Can you work these out from the model? Positions are in its coordinate system, mm. A direction names the side the tool comes from. Round coordinates to 2 decimals unless told otherwise and drop trailing zeros. Loops run counter-clockwise (first coordinate to the right, second up) from the corner with the lowest first, then second, coordinate; pieces in that order, holes last.
(1) If I drill on line 1 along Y through (x, z) = (-34, -19); line 2 along Y through (x, z) = (-16, -17); line 3 along Z through (x, y) = (-27.5, 6.5), over which ranges is the centre line in solid material (lowest first)?
(2) Which directions (+Z, -Z, +X, -X, +Y, -Y) give clear straight access to the entire face, cutting with the end or side of a thin tool? Please do faces 5 (the face through (8.428, 50.42, 1.107)), 6 (the face through (33, 2, 21)), 7 (the face through (39.05, 8.99, 8.67)).
(3) Thinking about a two-plate mould opening in Y: for faces 1 (the face through (0.33, 87.014, -7.493)), 2 (the face through (-14.75, 4.96, 35.58)), 3 (the face through (-3.874, 82.958, -5.052)), 4 (the face through (1, 0, 1)), which applies, released by +Y, released by -Y, zero draft, split by the parting line, or undercut?
(4) Will these pins go through, and if not, where does the flat tip stop? pin 1 Ø24 at (x, z) = (9.5, 15) entering from -Y; pin 2 Ø8 at (y, z) = (66, -3) entering from -X; pin 3 Ø12 at (y, z) = (57.5, 5) entering from +X; pin 4 Ø8 at (y, z) = (19, 11) entering from +X.
(5) I want a section at C-C on y = 23.5. Write out the boundary of the cut face in (x, z), plus the area to 3 significant figures.
(6) I want a section at D-D on z = 26. Write out the boundary of the cut face in (x, y), plus the area to 3 significant figures.
from build123d import *

# Parameters (mm, degrees)
SKETCH1_R           = 38.515
BOSS_EXTRUDE1_DEPTH = 10
SKETCH2_R           = 40
BOSS_EXTRUDE2_DEPTH = 2
BOSS_EXTRUDE3_START = -2
SKETCH3_R           = 40
BOSS_EXTRUDE3_DEPTH = 2
SKETCH4_R           = 6.366
BOSS_EXTRUDE4_DEPTH = 78
SKETCH5_R           = 7.5
BOSS_EXTRUDE5_DEPTH = 2
SKETCH6_R           = 8.5
BOSS_EXTRUDE6_DEPTH = 60
BOSS_EXTRUDE7_START = 4
SKETCH7_R           = 7.5
BOSS_EXTRUDE7_DEPTH = 4


with BuildPart() as part:
    # Sketch1 → Boss-Extrude1 (new body)
    with BuildSketch(Plane(origin=(0, 0, 0), x_dir=(1, 0, 0), z_dir=(0, 1, 0))):
        with Locations(Location((0, 0, 0), (0, 0, 270))):
            Circle(SKETCH1_R)
    extrude(amount=BOSS_EXTRUDE1_DEPTH)

    # Sketch2 → Boss-Extrude2 (add)
    with BuildSketch(Plane.XZ):
        with Locations(Location((0, 0, 0), (0, 0, 270))):
            Circle(SKETCH2_R)
    extrude(amount=-BOSS_EXTRUDE2_DEPTH)

    # Sketch3 → Boss-Extrude3 (add)
    with BuildSketch(Plane(origin=(0, 10, 0), x_dir=(1, 0, 0), z_dir=(0, 1, 0)).offset(BOSS_EXTRUDE3_START)):
        with Locations(Location((0, 0, 0), (0, 0, 90))):
            Circle(SKETCH3_R)
    extrude(amount=BOSS_EXTRUDE3_DEPTH)

    # Sketch4 → Boss-Extrude4 (add)
    with BuildSketch(Plane(origin=(0, 10, 0), x_dir=(1, 0, 0), z_dir=(0, 1, 0))):
        with Locations(Location((0, 0, 0), (0, 0, 270))):
            Circle(SKETCH4_R)
    extrude(amount=BOSS_EXTRUDE4_DEPTH)

    # Sketch5 → Boss-Extrude5 (add)
    with BuildSketch(Plane(origin=(0, 88, 0), x_dir=(1, 0, 0), z_dir=(0, 1, 0))):
        with Locations(Location((0, 0, 0), (0, 0, 270))):
            Circle(SKETCH5_R)
    extrude(amount=-BOSS_EXTRUDE5_DEPTH)

    # Sketch6 → Boss-Extrude6 (add)
    with BuildSketch(Plane(origin=(0, 80, 0), x_dir=(-1, 0, 0), z_dir=(0, -1, 0))):
        with Locations(Location((0, 0, 0), (0, 0, 90))):
            Circle(SKETCH6_R)
    extrude(amount=BOSS_EXTRUDE6_DEPTH)

    # Sketch7 → Boss-Extrude7 (add)
    with BuildSketch(Plane(origin=(0, 10, 0), x_dir=(1, 0, 0), z_dir=(0, 1, 0)).offset(BOSS_EXTRUDE7_START)):
        with Locations(Location((0, 0, 0), (0, 0, 270))):
            Circle(SKETCH7_R)
    extrude(amount=-BOSS_EXTRUDE7_DEPTH)


solid = part.part
Filled sheet:
1. line 1: y = 0 to 2, 8 to 10
1. line 2: y = 0 to 10
1. line 3: z = -26.97 to 26.97
2. face 5: +Y
2. face 6: none
2. face 7: +Y, -Y
3. face 1: zero draft
3. face 2: undercut
3. face 3: undercut
3. face 4: released by -Y
4. pin 1: stops at y = 0
4. pin 2: stops at x = -8.5
4. pin 3: stops at x = 8.5
4. pin 4: stops at x = 4.63
5. outline: circle Ø17 at (0, 0)
5. area: 227 mm2
6. outline: (-30.4, 0) - (30.4, 0) - (30.4, 2) - (28.41, 2) - (28.41, 8) - (30.4, 8) - (30.4, 10) - (-30.4, 10) - (-30.4, 8) - (-28.41, 8) - (-28.41, 2) - (-30.4, 2) - close
6. area: 584 mm2
